Source: CAD feature listing. Evaluate the final solid. Frame: model axes, mm. Face numbers are marked on the shaded views. Give positions to 0.01 mm unless a question says otherwise; leave off trailing zeros. Loops run counter-clockwise (first coordinate to the right, second up) from the corner with the lowest first, then second, coordinate; pieces in that order, holes last. Notation, with made-up numbers: (77.25, -33.5) - (107.25, -33.5) arc R20 cw to (107.25, -22.5) - close; hole circle Ø7 at (45, 28.5). An arc over 180 degrees is marked (long way). Write each question's results on one line, items separated by ' | '. Start each with the question number.
(1) Contact query for flat-ended pins moving along their axis: pin 1 (4 mm diameter, centred on x = 91.5, z = 5.5, fed in from +Y); pin 2 (5 mm diameter, centred on y = 82, z = 14, fed in from +X); pin 3 (10 mm diameter, centred on x = 89.5, z = 16.5, fed in from +Y). Output: stop coordinate, or through.
(2) Pull-direction query (Y, two-part tool) for the marked faces 1, 2 and 3; classes: pulls with the +Y half, pulls with the -Y half, needs draft (parallel to the pull), parting line crosses it, or undercut.
(3) Cut plane C-C on z = 25.5. Return the cut outline in (x, y).
(4) Cut plane A-A on y = 0. Return the cut outline in (x, z), then the cut area to 3 significant figures.
(5) Material intervals for line 1 along Y through (x, z) = (0, 7.5); line 2 along Y through (x, z) = (-35, 18.75); line 3 along Y through (x, z) = (34.5, 1.5), sorted ascending. Write a range as [from, to].
from build123d import *

# Parameters (mm, degrees)
F2_R     = 4
F3_DEPTH = 30.001


with BuildPart() as f1:
    # F0 (on Front) → F1 (revolve)
    with BuildSketch(Plane.XZ):
        with BuildLine():
            Line((87, 30), (87, 0))
            Line((87, 0), (92, 0))
            ThreePointArc((92, 0), (93.994377, 1.850134), (95.988754, 0))
            Line((95.988754, 0), (126.56137, 0))
            Line((126.56137, 0), (126.56137, 30))
            Line((126.56137, 30), (87, 30))
        make_face()
    revolve(axis=Axis((0, 0, 3.579337), (0, 0, 1)))

    # F2 (on face) → F3 (cut, through all)
    with BuildSketch(Plane.XY.offset(30)):
        with Locations((108.56137, 0)):
            Circle(F2_R)
        with Locations((0, 108.56137)):
            Circle(F2_R)
        with Locations((-108.56137, 0)):
            Circle(F2_R)
        with Locations((0, -108.56137)):
            Circle(F2_R)
    extrude(amount=-F3_DEPTH, mode=Mode.SUBTRACT)


solid = f1.part
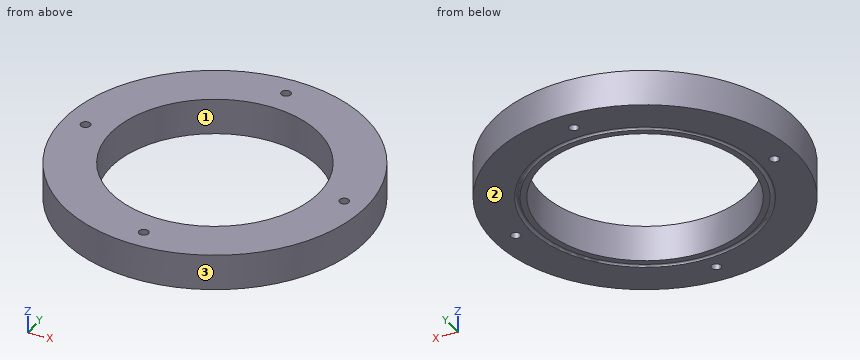
Ans:
1) pin 1: y = 89.48 | pin 2: x = 98.48 | pin 3: y = 94.22
2) face 1: undercut | face 2: needs draft | face 3: parting line crosses it
3) outline: circle Ø253.12 at (0, 0); hole circle Ø8 at (-108.56, 0); hole circle Ø174 at (0, 0); hole circle Ø8 at (0, -108.56); hole circle Ø8 at (0, 108.56); hole circle Ø8 at (108.56, 0)
4) outline: (-126.56, 0) - (-112.56, 0) - (-112.56, 30) - (-126.56, 30) - close; (-104.56, 0) - (-95.99, 0) arc R2 cw to (-92, 0) - (-87, 0) - (-87, 30) - (-104.56, 30) - close; (87, 0) - (92, 0) arc R2 cw to (95.99, 0) - (104.56, 0) - (104.56, 30) - (87, 30) - close; (112.56, 0) - (126.56, 0) - (126.56, 30) - (112.56, 30) - close | area: 1,880 mm^2
5) line 1: [-126.56, -112.56], [-104.56, -87], [87, 104.56], [112.56, 126.56] | line 2: [-121.63, -79.65], [79.65, 121.63] | line 3: [-121.77, -88.65], [-86.22, -79.87], [79.87, 86.22], [88.65, 121.77]
